Here's how the part is built. I have some questions about the finished solid (model axes, mm). A direction names the side the tool comes from. Give positions to 0.01 mm unless a question says otherwise; leave off trailing zeros. Order: outer loops, then holes, each group sorted by start corner. A loop starts at its lowest first (then second) coordinate and runs counter-clockwise, first axis right, second up.
from build123d import *

# Parameters (mm, degrees)
BOSS_EXTRUDE1_DEPTH     = 20
SKETCH2_R               = 2.4
CUT_EXTRUDE2_DEPTH      = 28.957878519
SKETCH3_R               = 3.1
CUT_EXTRUDE3_DEPTH      = 0.8
CUT_EXTRUDE4_REACH      = 34.348
CUT_EXTRUDE4_END_RADIUS = 6.25
SKETCH4_R               = 1.35
SKETCH5_R               = 1.35
CUT_EXTRUDE5_DEPTH      = 5
SKETCH6_R               = 2.4
CUT_EXTRUDE6_DEPTH      = 5
SKETCH7_R               = 3.1
CUT_EXTRUDE7_DEPTH      = 1


with BuildPart() as part:
    # Sketch1 → Boss-Extrude1 (new body)
    with BuildSketch(Plane(origin=(0, 0, 0), x_dir=(1, 0, 0), z_dir=(0, 1, 0))):
        with BuildLine():
            Line((7.077642728, 2.481324931), (16.7933357, 2.481324931))
            Line((16.7933357, 2.481324931), (16.7933357, 0.453397708))
            Line((16.7933357, 0.453397708), (16.7933357, -0.453397708))
            Line((16.7933357, -0.453397708), (16.7933357, -2.481324931))
            Line((16.7933357, -2.481324931), (7.077642728, -2.481324931))
            ThreePointArc((7.077642728, -2.481324931), (-7.5, 0), (7.077642728, 2.481324931))
        make_face()
        with BuildLine():
            ThreePointArc((6.109239102, 1.318975964), (-6.25, 0), (6.109239102, -1.318975964))
            ThreePointArc((6.109239102, -1.318975964), (6.25, 0), (6.109239102, 1.318975964))
        make_face(mode=Mode.SUBTRACT)
    boss_extrude1 = extrude(amount=BOSS_EXTRUDE1_DEPTH)

    # Sketch2 → Cut-Extrude2 (cut, through all)
    with BuildSketch(Plane.XY.offset(2.481324931)):
        with Locations((11.935489214, 14.25)):
            Circle(SKETCH2_R)
        with Locations((11.935489214, 5.75)):
            Circle(SKETCH2_R)
    extrude(amount=-CUT_EXTRUDE2_DEPTH, mode=Mode.SUBTRACT)

    # Sketch3 → Cut-Extrude3 (cut)
    with BuildSketch(Plane.XY.offset(2.481324931)):
        with Locations((11.935489214, 14.25)):
            Circle(SKETCH3_R)
        with Locations((11.935489214, 5.75)):
            Circle(SKETCH3_R)
    extrude(amount=-CUT_EXTRUDE3_DEPTH, mode=Mode.SUBTRACT)

    # Cut-Extrude4: up to this cylinder (the profile starts outside it)
    cut_extrude4_end = Plane(origin=(0, 10.443469, 0), z_dir=(0, -1, 0)) * Cylinder(CUT_EXTRUDE4_END_RADIUS, 82.196, mode=Mode.PRIVATE)
    # Sketch4 → Cut-Extrude4 (cut, up to the surface)
    with BuildSketch(Plane.ZY.offset(7.5), mode=Mode.PRIVATE) as cut_extrude4_sk1:
        with Locations((0, 10.443469374)):
            Circle(SKETCH4_R)
    cut_extrude4_tool1 = extrude(cut_extrude4_sk1.sketch, amount=-CUT_EXTRUDE4_REACH, mode=Mode.PRIVATE) - cut_extrude4_end
    cut_extrude4 = cut_extrude4_tool1.solids().sort_by_distance((-7.5, 10.443469, 0))[0]
    add(cut_extrude4, mode=Mode.SUBTRACT)

    # Mirror2: Boss-Extrude1, Cut-Extrude4 across plane
    add(boss_extrude1.mirror(Plane.ZX))
    add(cut_extrude4.mirror(Plane.ZX), mode=Mode.SUBTRACT)

    # Sketch5 → Cut-Extrude5 (cut)
    with BuildSketch(Plane.XY.offset(7.5)):
        with Locations((0, 10.938911234)):
            Circle(SKETCH5_R)
        with Locations((0, -10.702394235)):
            Circle(SKETCH5_R)
    extrude(amount=-CUT_EXTRUDE5_DEPTH, mode=Mode.SUBTRACT)

    # Sketch6 → Cut-Extrude6 (cut)
    with BuildSketch(Plane.XY.offset(2.481324931)):
        with Locations((11.935489214, -11.25)):
            Circle(SKETCH6_R)
        with Locations((11.935489214, -2.75)):
            Circle(SKETCH6_R)
    extrude(amount=-CUT_EXTRUDE6_DEPTH, mode=Mode.SUBTRACT)

    # Sketch7 → Cut-Extrude7 (cut)
    with BuildSketch(Plane.XY.offset(2.481324931)):
        with Locations((11.935489214, 5.75)):
            Circle(SKETCH7_R)
        with Locations((11.935489214, -2.75)):
            Circle(SKETCH7_R)
        with Locations((11.935489214, -11.25)):
            Circle(SKETCH7_R)
    extrude(amount=-CUT_EXTRUDE7_DEPTH, mode=Mode.SUBTRACT)


solid = part.part
Q1. I need wall thicknesses on L1, parallel to Y at x = -7, z = 0; L2, parallel to Y at x = 12.25, z = 2.25; L3, parallel to X at y = -1, z = 0. Which ranges of each line are inside material? Lowest first, please.
Filled sheet:
L1: y = -20 to -11.79, -9.09 to 9.09, 11.79 to 20
L2: y = -20 to -14.33, -8.17 to -5.83, 0.33 to 2.67, 8.83 to 11.17, 17.33 to 20
L3: x = -7.5 to -6.25, 6.25 to 10.29, 13.58 to 16.79
Q2. If we section it at A-A on z = 0: List the corners of the cut face in (x, y) for me, plus the area to 3 significant figures.
Filled sheet:
outline: (-7.5, -20) - (-6.25, -20) - (-6.25, -11.79) - (-7.5, -11.79) - close; (-7.5, -9.09) - (-6.25, -9.09) - (-6.25, 9.09) - (-7.5, 9.09) - close; (-7.5, 11.79) - (-6.25, 11.79) - (-6.25, 20) - (-7.5, 20) - close; (6.25, -20) - (16.79, -20) - (16.79, 20) - (6.25, 20) - close; hole circle Ø4.8 at (11.94, -11.25); hole circle Ø4.8 at (11.94, -2.75); hole circle Ø4.8 at (11.94, 5.75); hole circle Ø4.8 at (11.94, 14.25)
area: 393 mm2
Q3. Thinking about a two-plate mould opening in Z: for faces 1 (the face through (6.223, 0.28, -0.577)), 2 (the face through (-7.494, 0.28, 0.294)), 3 (the face through (13.23, -9.23, -0.47)), which applies, released by +Z, released by -Z, zero draft, split by the parting line, or undercut?
Filled sheet:
face 1: undercut
face 2: split by the parting line
face 3: zero draft
Q4. If we section it at B-B on x = 0: List the corners of the cut face in (y, z) for me, plus the area to 4 significant figures.
Filled sheet:
outline: (-20, -7.5) - (20, -7.5) - (20, -6.25) - (-20, -6.25) - close; (-20, 6.25) - (-12.05, 6.25) - (-12.05, 7.5) - (-20, 7.5) - close; (-9.35, 6.25) - (9.59, 6.25) - (9.59, 7.5) - (-9.35, 7.5) - close; (12.29, 6.25) - (20, 6.25) - (20, 7.5) - (12.29, 7.5) - close
area: 93.25 mm2
Q5. If we section it at C-C on y = -2.75: List the corners of the cut face in (x, z) for me, plus the area to 3 significant figures.
Filled sheet:
outline: (7.08, -2.48) - (9.54, -2.48) - (9.54, 1.48) - (8.84, 1.48) - (8.84, 2.48) - (7.08, 2.48) arc R7.5 ccw (long way) to start; (14.34, -2.48) - (16.79, -2.48) - (16.79, 2.48) - (15.04, 2.48) - (15.04, 1.48) - (14.34, 1.48) - close; hole circle Ø12.5 at (0, 0)
area: 75.6 mm2
Q6. If we section it at D-D on z = 4.5: List the corners of the cut face in (x, y) for me.
Filled sheet:
outline: (-6, -20) - (-4.34, -20) - (-4.34, 20) - (-6, 20) - close; (4.34, -20) - (6, -20) - (6, 20) - (4.34, 20) - close
Q7. For faces 4 (the face through (-6.809, 11.356, -0.995)), 5 (the face through (13.1, 0.3, 2.481)), 6 (the face through (9.48, -4.64, 1.99)), which set-ups out of +Z, -Z, +X, -X, +Y, -Y let a thin tool reach every point of the face, with its end or its side?
Filled sheet:
face 4: -X
face 5: +Z, +X, +Y, -Y
face 6: +Z
Q8. I'm going to push flat-ended pins straight in: P1, Ø8, axis at x = 11.94, y = 14.25, coming from the -Z side; P2, Ø5, axis at x = 8.5, y = 2.5, coming from the +Z side; P3, Ø3, axis at x = 12.5, y = -7, coming from the +Z side. Where does each tip first touch, or does it pass through?
Filled sheet:
P1: stops at z = -2.48
P2: stops at z = 4.5
P3: stops at z = 2.48
